from build123d import *

# Parameters (mm, degrees)
SKETCH2_R           = 15.25
SKETCH2_R_2         = 14.25
BOSS_EXTRUDE1_DEPTH = 10
BOSS_EXTRUDE2_START = -2
SKETCH4_R           = 14.25
BOSS_EXTRUDE2_DEPTH = 2
SKETCH5_R           = 12
CUT_EXTRUDE1_DEPTH  = 2
BOSS_EXTRUDE4_START = 15
SKETCH6_R           = 13
SKETCH6_R_2         = 12
BOSS_EXTRUDE4_DEPTH = 15
CUT_EXTRUDE3_DEPTH  = 34.017041055


with BuildPart() as part:
    # Sketch2 → Boss-Extrude1 (new body)
    with BuildSketch(Plane(origin=(0, 0, 0), x_dir=(1, 0, 0), z_dir=(0, 1, 0))):
        with Locations(Location((0, 0, 0), (0, 0, 270))):
            Circle(SKETCH2_R)
        with Locations(Location((0, 0, 0), (0, 0, 270))):
            Circle(SKETCH2_R_2, mode=Mode.SUBTRACT)
    extrude(amount=BOSS_EXTRUDE1_DEPTH)

    # Sketch4 → Boss-Extrude2 (add)
    with BuildSketch(Plane(origin=(0, 10, 0), x_dir=(1, 0, 0), z_dir=(0, 1, 0)).offset(BOSS_EXTRUDE2_START)):
        with Locations(Location((0, 0, 0), (0, 0, 270))):
            Circle(SKETCH4_R)
    extrude(amount=BOSS_EXTRUDE2_DEPTH)

    # Sketch5 → Cut-Extrude1 (cut)
    with BuildSketch(Plane(origin=(0, 10, 0), x_dir=(1, 0, 0), z_dir=(0, 1, 0))):
        with Locations(Location((0, 0, 0), (0, 0, 270))):
            Circle(SKETCH5_R)
    extrude(amount=-CUT_EXTRUDE1_DEPTH, mode=Mode.SUBTRACT)

    # Sketch6 → Boss-Extrude4 (add)
    with BuildSketch(Plane(origin=(0, 10, 0), x_dir=(1, 0, 0), z_dir=(0, 1, 0)).offset(BOSS_EXTRUDE4_START)):
        with Locations(Location((0, 0, 0), (0, 0, 270))):
            Circle(SKETCH6_R)
        with Locations(Location((0, 0, 0), (0, 0, 270))):
            Circle(SKETCH6_R_2, mode=Mode.SUBTRACT)
    extrude(amount=-BOSS_EXTRUDE4_DEPTH)

    # Sketch7 → Cut-Extrude3 (cut, through all)
    with BuildSketch(Plane(origin=(0, 25, 0), x_dir=(1, 0, 0), z_dir=(0, 1, 0))):
        with BuildLine():
            ThreePointArc((-1.6, 12.901162738), (0, 13), (1.6, 12.901162738))
            Line((1.6, 12.901162738), (1.6, 13.5))
            Line((1.6, 13.5), (-1.6, 13.5))
            Line((-1.6, 13.5), (-1.6, 12.901162738))
        make_face()
        with BuildLine():
            ThreePointArc((-1.6, 11.892854998), (0, 12), (1.6, 11.892854998))
            Line((1.6, 11.892854998), (1.6, 12.901162738))
            ThreePointArc((1.6, 12.901162738), (0, 13), (-1.6, 12.901162738))
            Line((-1.6, 12.901162738), (-1.6, 11.892854998))
        make_face()
        with BuildLine():
            ThreePointArc((1.6, -12.901162738), (0.801524922, -12.975267157), (0, -13))
            Line((0, -13), (0, -13.5))
            Line((0, -13.5), (1.6, -13.5))
            Line((1.6, -13.5), (1.6, -12.901162738))
        make_face()
        with BuildLine():
            Line((0, -13.5), (0, -13))
            ThreePointArc((0, -13), (-0.801524922, -12.975267157), (-1.6, -12.901162738))
            Line((-1.6, -12.901162738), (-1.6, -13.5))
            Line((-1.6, -13.5), (0, -13.5))
        make_face()
        with BuildLine():
            Line((0, -13), (0, -12))
            ThreePointArc((0, -12), (-0.801791752, -11.973183787), (-1.6, -11.892854998))
            Line((-1.6, -11.892854998), (-1.6, -12.901162738))
            ThreePointArc((-1.6, -12.901162738), (-0.801524922, -12.975267157), (0, -13))
        make_face()
        with BuildLine():
            ThreePointArc((1.6, -11.892854998), (0.801791752, -11.973183787), (0, -12))
            Line((0, -12), (0, -13))
            ThreePointArc((0, -13), (0.801524922, -12.975267157), (1.6, -12.901162738))
            Line((1.6, -12.901162738), (1.6, -11.892854998))
        make_face()
    extrude(amount=-CUT_EXTRUDE3_DEPTH, mode=Mode.SUBTRACT)


solid = part.part
Could you check a few things on this model? Use its own coordinates, in mm. A direction names the side the tool comes from. Round coordinates to 2 decimals unless told otherwise and drop trailing zeros. Order: outer loops, then holes, each group sorted by start corner. A loop starts at its lowest first (then second) coordinate and runs counter-clockwise, first axis right, second up.
Q1. Which directions (+Z, -Z, +X, -X, +Y, -Y) give clear straight access to the entire face, cutting with the end or side of a thin tool? Please do faces 1 (the face through (-1.6, 16.6, 12.5)), 2 (the face through (-11.23, 10, -6.85)), 3 (the face through (-13.91, 3.94, -3.09)), 4 (the face through (-13, 18, 0)).
Geometry says:
face 1: +Y, -Y
face 2: +Y
face 3: -Y
face 4: -X, +Y
Q2. Thinking about a two-plate mould opening in X: for faces 5 (the face through (-14.887, 4.93, -3.306)), 6 (the face through (1.6, 16.6, -12.5)), 7 (the face through (14, 0, -5)), which applies, released by +X, released by -X, zero draft, split by the parting line, or undercut?
Geometry says:
face 5: split by the parting line
face 6: undercut
face 7: zero draft
Q3. Imagine slicing it at B-B, the plane y = 11.5. List the corners of the cut face in (x, z) for me.
Geometry says:
outline: (-1.6, -12.9) - (-1.6, -11.89) arc R12 cw to (-1.6, 11.89) - (-1.6, 12.9) arc R13 ccw to start; (1.6, -12.9) arc R13 ccw to (1.6, 12.9) - (1.6, 11.89) arc R12 cw to (1.6, -11.89) - close
Q4. Imagine slicing it at C-C, the plane x = 0. List the corners of the cut face in (y, z) for me.
Geometry says:
outline: (0, -15.25) - (10, -15.25) - (10, -13.5) - (8, -13.5) - (8, -14.25) - (0, -14.25) - close; (0, 14.25) - (8, 14.25) - (8, 13.5) - (10, 13.5) - (10, 15.25) - (0, 15.25) - close
Q5. I'm going to push flat-ended pins straight in: P1, Ø5, axis at x = 1, y = 15.5, coming from the -Z side; P2, Ø6, axis at y = 14.5, z = 8.5, coming from the -X side; P3, Ø2, axis at x = 0.5, y = 21.5, coming from the +Z side; P4, Ø1.3, axis at y = 20, z = 12.5, coming from the -X side. Where does each tip first touch, or does it pass through?
Geometry says:
P1: stops at z = -12.9
P2: stops at x = -11.78
P3: passes through
P4: stops at x = -5.35
Q6. Imagine slicing it at D-D, the plane y = 2.25. List the corners of the cut face in (x, z) for me.
Geometry says:
outline: circle Ø30.5 at (0, 0); hole circle Ø28.5 at (0, 0)
Q7. Imagine slicing it at A-A, the plane z = 0. List the corners of the cut face in (x, y) for me, then the cut area to 3 significant figures.
Geometry says:
outline: (-15.25, 0) - (-14.25, 0) - (-14.25, 8) - (-12, 8) - (-12, 25) - (-13, 25) - (-13, 10) - (-15.25, 10) - close; (12, 8) - (14.25, 8) - (14.25, 0) - (15.25, 0) - (15.25, 10) - (13, 10) - (13, 25) - (12, 25) - close
area: 59.0 mm2
Q8. Please list where these lines run through material, in increasing order: probe 1 along X at (y, z) = (2.5, 0); probe 2 along Y at (x, z) = (11, -5.5); probe 3 along X at (y, z) = (18, -9).
Geometry says:
probe 1: x = -15.25 to -14.25, 14.25 to 15.25
probe 2: y = 8 to 25
probe 3: x = -9.38 to -7.94, 7.94 to 9.38
